from build123d import *

# Parameters (mm, degrees)
ESBO_O1_W                = 50
ESBO_O1_H                = 9.53
RESSALTO_EXTRUS_O1_DEPTH = 30
ESBO_O2_R                = 3
CORTE_EXTRUS_O1_DEPTH    = 40.340884904
ESBO_O4_W                = 30
ESBO_O4_H                = 9.53
RESSALTO_EXTRUS_O3_DEPTH = 60.01
ESBO_O5_W                = 30
ESBO_O5_H                = 9.53
RESSALTO_EXTRUS_O4_DEPTH = 33
ESBO_O6_R                = 2.5
CORTE_EXTRUS_O2_DEPTH    = 10
CORTE_EXTRUS_O3_REACH    = 92.651
ESBO_O7_R                = 3


with BuildPart() as part:
    # Esboço1 → Ressalto-extrusão1 (new body)
    with BuildSketch(Plane.XY):
        Rectangle(ESBO_O1_W, ESBO_O1_H)
    extrude(amount=RESSALTO_EXTRUS_O1_DEPTH)

    # Esboço2 → Corte-extrusão1 (cut, through all)
    with BuildSketch(Plane.XY.offset(30)):
        with Locations((-13, 0)):
            Circle(ESBO_O2_R)
    extrude(amount=-CORTE_EXTRUS_O1_DEPTH, mode=Mode.SUBTRACT)

    # Esboço4 → Ressalto-extrusão3 (add)
    with BuildSketch(Plane(origin=(25, 0, 0), x_dir=(0, 0, -1), z_dir=(1, 0, 0))):
        with Locations((-15, 0)):
            Rectangle(ESBO_O4_W, ESBO_O4_H)
    extrude(amount=RESSALTO_EXTRUS_O3_DEPTH)

    # Esboço5 → Ressalto-extrusão4 (add)
    with BuildSketch(Plane.ZY.offset(25)):
        with Locations((15, 0)):
            Rectangle(ESBO_O5_W, ESBO_O5_H)
    extrude(amount=RESSALTO_EXTRUS_O4_DEPTH)

    # Esboço6 → Corte-extrusão2 (cut)
    with BuildSketch(Plane.XY.offset(30)):
        with Locations((-31, 0)):
            Circle(ESBO_O6_R)
        with Locations((58.01, 0)):
            Circle(ESBO_O6_R)
    extrude(amount=-CORTE_EXTRUS_O2_DEPTH, mode=Mode.SUBTRACT)

    # Esboço7 → Corte-extrusão3 (cut, up to next)
    with BuildSketch(Plane(origin=(0, 4.765, 0), x_dir=(1, 0, 0), z_dir=(0, 1, 0)), mode=Mode.PRIVATE) as corte_extrus_o3_sk1:
        with Locations(Location((13.505, -15, 0), (0, 0, 270))):
            Circle(ESBO_O7_R)
    corte_extrus_o3_tool1 = extrude(corte_extrus_o3_sk1.sketch, amount=-CORTE_EXTRUS_O3_REACH, mode=Mode.PRIVATE) & part.part
    add(corte_extrus_o3_tool1.solids().sort_by_distance((13.505, 4.765, 15))[0], mode=Mode.SUBTRACT)


solid = part.part
CAD build for the part. Positions are in the model's coordinates, mm. A direction names the side the tool comes from. Coordinates: 2 decimals unless noted, no trailing zeros. Write each loop counter-clockwise with the first axis right and the second up, starting at its lowest first coordinate (ties: lowest second). Pieces come first, ordered by that corner, then holes. Notation, with made-up numbers: M 28.5,66.25 L 74.5,66.25 A12 ccw 74.5,85.25 Z; hole C 1.25,43 d10. An arc over 180 degrees is marked long. Answer as a JSON object with one key per item and string values. Group by question number.
1) Saw through at B-B (z = 15). Write the cut outline in (x, y) (3 decimals).
2) Wall check: line 1 (Y direction, x = 58.01, z = 27.5) (3 decimals); line 2 (X direction, y = -0.5, z = 17.75); line 3 (X direction, y = -2, z = 24). Give the ranges that are in metal, low to high. Write a range as from..to.
3) Mould opens along Y. For faces 1 (the face through (58, 0, 20)), 2 (the face through (15, -4.765, 11)), 3 (the face through (60.3, -1, 25.1)), 4 (the face through (85.01, 0, 15)) say: +Y half, -Y half, draft (parallel to the pull), parting line (faces both ways), or undercut.
4) Saw through at C-C (x = -13). Write the cut outline in (y, z) (3 decimals), plus the area to 3 significant figures.
5) Saw through at D-D (z = 21.5). Write the cut outline in (x, y) (3 decimals).
6) Tool access for faces 5 (the face through (-33.5, 0.1, 25.1)), 6 (the face through (15, 0, 30)): list every direction of +Z, -Z, +X, -X, +Y, -Y with a clear straight run to the whole face (end or side of a thin tool).
7) Pin check, flat tips, straight feed: pin 1 Ø2.5 at (x, y) = (57.5, 0.5) entering from +Z; pin 2 Ø5 at (x, z) = (13.505, 15) entering from +Y. Stop position of each tip, or through.
8) Saw through at A-A (y = 0). Write the cut outline in (x, z) (3 decimals), plus the area to 3 significant figures.
Values follow:
{
 "1": {"outline": "M -58,-4.765 L 10.505,-4.765 L 10.505,4.765 L -58,4.765 Z; M 16.505,-4.765 L 85.01,-4.765 L 85.01,4.765 L 16.505,4.765 Z; hole C -13,0 d6"},
 "2": {"line 1": "y = -4.765..-2.5, 2.5..4.765", "line 2": "x = -58..-15.96, -10.04..12.31, 14.7..85.01", "line 3": "x = -58..-32.5, -29.5..-15.24, -10.76..56.51, 59.51..85.01"},
 "3": {"face 1": "undercut", "face 2": "-Y half", "face 3": "undercut", "face 4": "draft"},
 "4": {"outline": "M -4.765,0 L -3,0 L -3,30 L -4.765,30 Z; M 3,0 L 4.765,0 L 4.765,30 L 3,30 Z", "area": "106 mm2"},
 "5": {"outline": "M -58,-4.765 L 85.01,-4.765 L 85.01,4.765 L -58,4.765 Z; hole C -31,0 d5; hole C -13,0 d6; hole C 58.01,0 d5"},
 "6": {"face 5": "+Z", "face 6": "+Z, +X, -X, +Y, -Y"},
 "7": {"pin 1": "stops at z = 20", "pin 2": "passes through"},
 "8": {"outline": "M -58,0 L -16,0 L -16,30 L -28.5,30 L -28.5,20 L -33.5,20 L -33.5,30 L -58,30 Z; M -10,0 L 85.01,0 L 85.01,30 L 60.51,30 L 60.51,20 L 55.51,20 L 55.51,30 L -10,30 Z; hole C 13.505,15 d6", "area": "3,980 mm2"}
}
